Check sheet for the modelled part. Datum: model origin and axes. Units: mm. A direction names the side the tool comes from. Coordinates: 2 decimals unless noted, no trailing zeros. Write each loop counter-clockwise with the first axis right and the second up, starting at its lowest first coordinate (ties: lowest second). Pieces come first, ordered by that corner, then holes. Notation, with made-up numbers: M 66.25,-19.5 L 71.25,-19.5 A20 ccw 71.25,-1.5 Z; hole C 34.25,-20.5 d7. An arc over 180 degrees is marked long. Answer as CSV lines item,"result". Start each with the question number.
Q1. Thickness scan on line 1 along Z through (x, y) = (-19.5, 6.5); line 2 along X through (y, z) = (6, 2.5); line 3 along Y through (x, z) = (-1.5, 6). Record the ranges inside material, lowest first. Write a range as from..to.
Q2. Depth check by flat-ended pin: pin 1 Ø1.5 at (x, z) = (5.5, 3.5) entering from -Y; pin 2 Ø3 at (x, y) = (-17.5, -6) entering from -Z; pin 3 Ø3.5 at (x, y) = (-17.32, -10) entering from -Z; pin 4 Ø6.5 at (x, y) = (0, 20) entering from +Z. Enter the tip coordinate at first touch or a pass-through.
Q3. Sectioned sample at B-B, the plane y = 0. Record the cut outline in (x, z), then the cut area to 3 significant figures.
Q4. Sectioned sample at D-D, the plane y = -10. Record the cut outline in (x, z), then the cut area to 3 significant figures.
Q5. Sectioned sample at A-A, the plane x = 0. Record the cut outline in (y, z).
Q6. Sectioned sample at C-C, the plane y = 20. Record the cut outline in (x, z), then the cut area to 3 significant figures.
Q7. Mould release check, pull along Y, two halves, no side actions. Record for faces 1 (the flat face through (0, 11, 2)), 2 (the cylindrical face through (-6.37, -28.7, 6.48)), 3 (the cylindrical face through (18.396, -8.314, 6.521)): pulls with the +Y half, pulls with the -Y half, needs draft (parallel to the pull), parting line crosses it, or undercut.
Q8. Access from +Z, -Z, +X, -X, +Y, -Y to the whole of each face (thin tool, end or side, straight path). Record for faces 4 (the flat face through (11.5, 0, 2)), 5 (the flat face through (-11.5, 0, 2)), 6 (the flat face through (0, -11, 2)).
from build123d import *

# Parameters (mm, degrees)
SKETCH1_W           = 23
SKETCH1_H           = 22
BOSS_EXTRUDE1_DEPTH = 5
SKETCH3_R           = 29.4
BOSS_EXTRUDE2_DEPTH = 3
SKETCH4_R           = 2
CUT_EXTRUDE1_DEPTH  = 3


with BuildPart() as part:
    # Sketch1 → Boss-Extrude1 (new body)
    with BuildSketch(Plane.XY):
        Rectangle(SKETCH1_W, SKETCH1_H)
    extrude(amount=BOSS_EXTRUDE1_DEPTH)

    # Sketch3 → Boss-Extrude2 (add)
    with BuildSketch(Plane.XY.offset(5)):
        Circle(SKETCH3_R)
    extrude(amount=BOSS_EXTRUDE2_DEPTH)

    # Sketch4 → Cut-Extrude1 (cut)
    with BuildSketch(Plane.XY.offset(8)):
        with Locations((0, 20)):
            Circle(SKETCH4_R)
        with Locations((17.320508076, -10)):
            Circle(SKETCH4_R)
        with Locations((-17.320508076, -10)):
            Circle(SKETCH4_R)
    extrude(amount=-CUT_EXTRUDE1_DEPTH, mode=Mode.SUBTRACT)


solid = part.part
Output:
1,line 1,"z = 5..8"
1,line 2,"x = -11.5..11.5"
1,line 3,"y = -29.36..18.68, 21.32..29.36"
2,pin 1,"stops at y = -11"
2,pin 2,"stops at z = 5"
2,pin 3,"passes through"
2,pin 4,"stops at z = 8"
3,outline,"M -29.4,5 L -11.5,5 L -11.5,0 L 11.5,0 L 11.5,5 L 29.4,5 L 29.4,8 L -29.4,8 Z"
3,area,"291 mm^2"
4,outline,"M -27.65,5 L -19.32,5 L -19.32,8 L -27.65,8 Z; M -15.32,5 L -11.5,5 L -11.5,0 L 11.5,0 L 11.5,5 L 15.32,5 L 15.32,8 L -15.32,8 Z; M 19.32,5 L 27.65,5 L 27.65,8 L 19.32,8 Z"
4,area,"257 mm^2"
5,outline,"M -29.4,5 L -11,5 L -11,0 L 11,0 L 11,5 L 18,5 L 18,8 L -29.4,8 Z; M 22,5 L 29.4,5 L 29.4,8 L 22,8 Z"
6,outline,"M -21.55,5 L -2,5 L -2,8 L -21.55,8 Z; M 2,5 L 21.55,5 L 21.55,8 L 2,8 Z"
6,area,"117 mm^2"
7,face 1,"pulls with the +Y half"
7,face 2,"parting line crosses it"
7,face 3,"undercut"
8,face 4,"-Z, +X, +Y, -Y"
8,face 5,"-Z, -X, +Y, -Y"
8,face 6,"-Z, +X, -X, -Y"
